Solid Edge part; units mm, degrees
sketch "Sketch1" plane through (0, 0, 0) normal (0, -1, 0) x (1, 0, 0)
  line L0 (-30, 0) -> (-30, 100)
  line L1 (-30, 100) -> (30, 100)
  line L2 (30, 100) -> (30, 0)
  line L3 (-30, 0) -> (30, 0)
  line L4 (-30, 0) -> (-90, 0)
  arc A0 (-90, 0) -> (-90, -50) centre (-90, -25) ccw
  line L5 (-90, -50) -> (0, -50)
  line L6 (90, -50) -> (0, -50)
  arc A1 (90, 0) -> (90, -50) centre (90, -25) cw
  line L7 (30, 0) -> (90, 0)
  line L8 (30, 0) -> (0, 0)
  line L9 (0, 0) -> (-30, 0)
  circle A2 centre (-90, -25) radius 10
  circle A3 centre (90, -25) radius 10
extrude "Protrusion1" add sketch "Sketch1" against normal blind 30
sketch "Sketch2" plane through (0, 0, 25) normal (0, -1, 0) x (1, 0, 0)
  circle A0 centre (0, 75) radius 30
extrude "ExtrudedCutout_1" cut sketch "Sketch2" against normal blind 30
sketch "Sketch3" plane through (0, 0, 25) normal (0, -1, 0) x (1, 0, 0)
  circle A0 centre (0, 75) radius 30
  circle A1 centre (0, 75) radius 15
extrude "ExtrudedProtrusion_2" add sketch "Sketch3" against normal blind 30 and the other way blind 10
fillet "Round_1" radius 10 2 edges at (30, 15, 0) (-30, 15, 0)
sketch "Sketch4" plane through (30, 0, 0) normal (1, 0, 0) x (0, 1, 0)
  line L0 (0, 30) -> (-79.7565, 14.5434)
  line L1 (0, -50) -> (0, 30)
  line L2 (0, -50) -> (-79.7565, -34.5434)
  arc A0 (-79.7565, -34.5433) -> (-79.7565, 14.5433) centre (-75, -10) cw
  circle A1 centre (-75, -10) radius 12.5
extrude "ExtrudedProtrusion_3" add sketch "Sketch4" against normal blind 15
mirror "Mirror1" about plane through (0, 0, 0) normal (1, 0, 0) of "ExtrudedProtrusion_3"
The listing builds one solid part. Answer for the finished solid, in the listing's coordinates (mm). A direction names the side the tool comes from. Give positions to 0.01 mm unless a question says otherwise; leave off trailing zeros. Loops run counter-clockwise (first coordinate to the right, second up) from the corner with the lowest first, then second, coordinate; pieces in that order, holes last. Notation, with made-up numbers: M 65.25,13 L 86.25,13 A8 cw 86.25,25 Z; hole C -11,-9.5 d3. An arc over 180 degrees is marked long. One line per item, written item: value.
Q1. A cutting plane is placed at A-A on x = 0. Determine the outline of the cut face in (y, z).
Working result:
outline: M -10,70 L 0,70 L 0,-50 L 30,-50 L 30,85 L -10,85 Z; M -10,115 L 30,115 L 30,130 L -10,130 Z
Q2. Find the intervals of material crossed by line 1 (X direction, y = -26.5, z = -26); line 2 (Z direction, x = -90, y = 7.5); line 3 (Y direction, x = -4, z = -2), in increasing order. Write a range as from..to.
Working result:
line 1: x = -30..-15, 15..30
line 2: z = -50..-35, -15..0
line 3: y = 0..30
Q3. A cutting plane is placed at D-D on y = -77. Determine the outline of the cut face in (x, z), then the cut area to 3 significant figures.
Working result:
outline: M -30,-35.08 L -15,-35.08 L -15,-22.34 L -30,-22.34 Z; M -30,2.34 L -15,2.34 L -15,15.08 L -30,15.08 Z; M 15,-35.08 L 30,-35.08 L 30,-22.34 L 15,-22.34 Z; M 15,2.34 L 30,2.34 L 30,15.08 L 15,15.08 Z
area: 764 mm^2
Q4. For faces 1 (the face through (30, -21, 9)), 2 (the face through (-3.905, 5.276, 129.745)), 3 (the face through (15, -40, -11)), determine the directions among +Z, -Z, +X, -X, +Y, -Y from which every point of the face is accessible in a straight line to the end or side of a thin tool.
Working result:
face 1: +Z, +X, -Y
face 2: -Y
face 3: -Z, -Y
Q5. Determine the mould class of faces 4 (the face through (114.994, 14.79, -25.55)), 5 (the face through (-100, 15, -25)), 6 (the face through (0, 0, 26)), 7 (the face through (-32.85, 15.21, 3.01)) for opening direction Z: +Z half, -Z half, draft (parallel to the pull), parting line (faces both ways), or undercut.
Working result:
face 4: parting line
face 5: undercut
face 6: undercut
face 7: +Z half
Q6. Flat-ended cylindrical pins translate along their axes: P1, Ø10, axis at x = -18, z = 1, coming from the -Y side; P2, Ø24, axis at y = -49, z = 1.5, coming from the +X side; P3, Ø5, axis at x = 18, z = 67.5, coming from the -Y side. Find the tip coordinate at first contact, or state that the pin passes through.
Working result:
P1: stops at y = -99.27
P2: stops at x = 30
P3: stops at y = 0
Q7. A cutting plane is placed at C-C on y = -13. Determine the outline of the cut face in (x, z), then the cut area to 3 significant figures.
Working result:
outline: M -30,-47.48 L -15,-47.48 L -15,27.48 L -30,27.48 Z; M 15,-47.48 L 30,-47.48 L 30,27.48 L 15,27.48 Z
area: 2,250 mm^2
Q8. A cutting plane is placed at B-B on z = -10. Determine the outline of the cut face in (x, y).
Working result:
outline: M -110,0 L -30,0 L -30,-62.5 L -15,-62.5 L -15,0 L 15,0 L 15,-62.5 L 30,-62.5 L 30,0 L 110,0 L 110,30 L -110,30 Z; M -30,-100 L -15,-100 L -15,-87.5 L -30,-87.5 Z; M 15,-100 L 30,-100 L 30,-87.5 L 15,-87.5 Z
